Can you work these out from the model? Positions are in its coordinate system, mm. Face numbers are marked on the shaded views. A direction names the side the tool comes from. Give positions to 0.01 mm unless a question says otherwise; leave off trailing zeros. One line per item, written item: value. Start each with the question number.
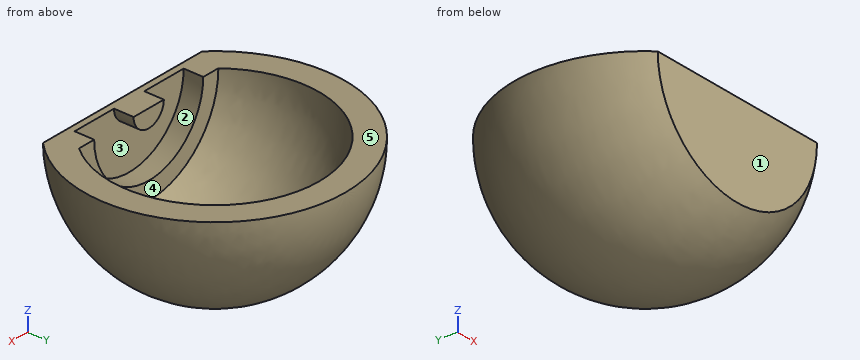
from build123d import *

# Parameters (mm, degrees)
REVOLUTION_ANGLE = 180


with BuildPart() as part:
    # Sketch → Revolution (revolve)
    with BuildSketch(Plane.XY):
        with BuildLine():
            ThreePointArc((70.710678, -70.710678), (92.387953, 38.268343), (0, 100))
            Line((0, 100), (0, 80))
            ThreePointArc((61.874285, -50.710678), (72.307864, 34.228247), (0, 80))
            Line((61.874285, -50.710678), (48.437142, -50.710678))
            Line((48.437142, -50.710678), (48.437142, -65.710678))
            Line((48.437142, -65.710678), (13.437142, -65.710678))
            Line((13.437142, -65.710678), (13.437142, -50.710678))
            Line((13.437142, -50.710678), (0, -50.710678))
            Line((0, -50.710678), (0, -70.710678))
            Line((70.710678, -70.710678), (0, -70.710678))
        make_face()
    revolve(axis=Axis((0, 0, 0), (0, 1, 0)), revolution_arc=REVOLUTION_ANGLE)


solid = part.part
Q1. I need wall thicknesses on line 1 along Y through (x, z) = (11, -38.5); line 2 along X through (y, z) = (-32.5, -43.5); line 3 along Y through (x, z) = (-20, -11.5). Which ranges of each line are inside material? Lowest first, please.
Q2. Which directions (+Z, -Z, +X, -X, +Y, -Y) give clear straight access to the entire face, cutting with the end or side of a thin tool? Please do the marked faces 3, 4 and 5.
Q3. If we mould it in two halves opening along X, with no side actions, what happens to the marked faces 1 and 2? For each: released by +X, released by -X, zero draft, split by the parting line, or undercut.
Q4. For P1, Ø8, axis at x = -33.5, y = 45.5, coming from the -Z side; P2, Ø4, axis at x = 4.5, z = -6, coming from the +Y side; P3, Ø1, axis at y = 51.5, z = -28.5, coming from the +X side, each with a flat end and sliding along its axis, tell me the tip position at first contact or that it passes through.
Response:
1. line 1: -70.71 to -65.71, 69.26 to 91.63
1. line 2: -83.97 to -58.75, 58.75 to 83.97
1. line 3: -70.71 to -65.71, 76.6 to 97.3
2. face 3: none
2. face 4: +Z
2. face 5: +Z, +X, -X, +Y, -Y
3. face 1: zero draft
3. face 2: undercut
4. P1: z = -85.11
4. P2: y = 99.85
4. P3: x = 81.2
